Verification items for the finished model (mm, model axes). A direction names the side the tool comes from. Coordinates: 2 decimals unless noted, no trailing zeros. Loops run counter-clockwise (first coordinate to the right, second up) from the corner with the lowest first, then second, coordinate; pieces in that order, holes last. Notation, with made-up numbers: (0, 71.5) - (53, 71.5) arc R25 ccw to (53, 94.5) - close; hole circle Ø10 at (8, 85). An arc over 180 degrees is marked (long way). Answer as CSV lines item,"result". Start each with the question number.
1. Set-up check for faces 5 (the flat face through (0, 35, 0)), 6 (the flat face through (-9, 23, 2)), 7 (the flat face through (-4.5, 3, 0)), 8 (the flat face through (-12, 10, 3)): record each of +Z, -Z, +X, -X, +Y, -Y from which the full face is reachable in a straight line by a thin tool's end or side.
2. Cross-section at D-D (y = 39). Enter the section's corners in (x, z), plus the area to 3 significant figures.
3. Cross-section at A-A (z = 5). Enter the section's corners in (x, y), plus the area to 3 significant figures.
4. Cross-section at B-B (y = 5.5). Enter the section's corners in (x, z).
5. Gauge pin test, flat ends, axial feed: P1, Ø3.5, axis at x = 12, y = 14.5, coming from the +Z side; P2, Ø3, axis at x = 2.5, z = -4.5, coming from the -Y side. Record the tip position at first contact, or that the pin passes through.
6. Material ranges on line 1 (X direction, y = 5, z = 4); line 2 (X direction, y = 39, z = -4); line 3 (X direction, y = 18, z = 3.5), recorded low to high. Write a range as [from, to].
7. Release check for a two-part mould opening along X. For faces 1 (the flat face through (-20, 20, -1)), 2 (the flat face through (-16, 23, 2)), 3 (the cylindrical face through (0.239, 19.358, 0.084)), 4 (the flat face through (18, 10, 6)) record: pulls with the +X half, pulls with the -X half, needs draft (parallel to the pull), parting line crosses it, or undercut.
8. Cross-section at C-C (z = -3). Enter the section's corners in (x, y).
```python
from build123d import *

# Parameters (mm, degrees)
SKETCH002_W          = 40
SKETCH002_H          = 12
POCKET_DEPTH         = 50.001
POCKET001_DEPTH      = 12.001
POCKET001_DEPTH_BACK = 0.001


with BuildPart() as part:
    # AdditivePipe: sweep along a path in Sketch
    with BuildLine(Plane.YZ) as additivepipe_path:
        Line((0, 0), (20, 0))
        Line((20, 0), (50, -12))
    # Sketch001 → AdditivePipe (sweep)
    with BuildSketch(Plane.XZ):
        Polygon((-20, 6), (-20, -6), (20, -6), (20, 6), (16, 6), (16, 3), (9, 3), (9, 6), (-9, 6), (-9, 3), (-16, 3), (-16, 6), align=None)
    sweep(path=additivepipe_path.line)

    # Sketch002 → Pocket (cut, through all)
    with BuildSketch(Plane.XZ):
        with Locations((0, -12)):
            Rectangle(SKETCH002_W, SKETCH002_H)
    extrude(amount=-POCKET_DEPTH, mode=Mode.SUBTRACT)

    # Sketch003 (on Face9 of Pocket) → Pocket001 (cut, two sides)
    with BuildSketch(Plane(origin=(0, 0, 6), x_dir=(-1, 0, 0), z_dir=(0, 0, 1))) as pocket001_sk:
        with BuildLine():
            Line((-4.5, 0), (4.5, 0))
            Line((4.5, 0), (4.5, -7))
            ThreePointArc((-4.5, -7), (0, -19.361903), (4.5, -7))
            Line((-4.5, 0), (-4.5, -7))
        make_face()
    extrude(amount=-POCKET001_DEPTH, mode=Mode.SUBTRACT)
    extrude(pocket001_sk.sketch, amount=POCKET001_DEPTH_BACK, mode=Mode.SUBTRACT)


solid = part.part
```
Values follow:
1,face 5,"+Z, +X, -X, +Y"
1,face 6,"+Z, +Y"
1,face 7,"+Z, -Z, -Y"
1,face 8,"+Z, +Y, -Y"
2,outline,"(-20, -6) - (20, -6) - (20, -1.6) - (16, -1.6) - (16, -4.6) - (9, -4.6) - (9, -1.6) - (-9, -1.6) - (-9, -4.6) - (-16, -4.6) - (-16, -1.6) - (-20, -1.6) - close"
2,area,"134 mm²"
3,outline,"(-20, 0) - (-16, 0) - (-16, 22.5) - (-20, 22.5) - close; (-9, 0) - (-4.5, 0) - (-4.5, 7) arc R7 cw (long way) to (4.5, 7) - (4.5, 0) - (9, 0) - (9, 22.5) - (-9, 22.5) - close; (16, 0) - (20, 0) - (20, 22.5) - (16, 22.5) - close"
3,area,"378 mm²"
4,outline,"(-20, -6) - (-4.5, -6) - (-4.5, 6) - (-9, 6) - (-9, 3) - (-16, 3) - (-16, 6) - (-20, 6) - close; (4.5, -6) - (20, -6) - (20, 6) - (16, 6) - (16, 3) - (9, 3) - (9, 6) - (4.5, 6) - close"
5,P1,"stops at z = 3"
5,P2,"stops at y = 18.11"
6,line 1,"x = [-20, -16], [-9, -4.5], [4.5, 9], [16, 20]"
6,line 2,"x = [-20, -16], [-9, 9], [16, 20]"
6,line 3,"x = [-20, -16], [-9, -4.15], [4.15, 9], [16, 20]"
7,face 1,"pulls with the -X half"
7,face 2,"undercut"
7,face 3,"undercut"
7,face 4,"needs draft"
8,outline,"(-20, 0) - (-4.5, 0) - (-4.5, 7) arc R7 cw (long way) to (4.5, 7) - (4.5, 0) - (20, 0) - (20, 42.5) - (16, 42.5) - (16, 35) - (9, 35) - (9, 42.5) - (-9, 42.5) - (-9, 35) - (-16, 35) - (-16, 42.5) - (-20, 42.5) - close"
